Input: part model. Units: mm. Frame: model coordinates. Coordinates: 2 decimals unless noted, no trailing zeros. Order: outer loops, then holes, each group sorted by start corner. A loop starts at its lowest first (then second) coordinate and runs counter-clockwise, first axis right, second up. Notation, with made-up numbers: (23, -34) -> (29, -34) arc R34 cw to (29, 4) -> close; hole circle Ø8 at (-10, -23). An arc over 180 degrees is marked (long way). Answer as CSV lines item,"result".
from build123d import *

# Parameters (mm, degrees)
SKETCH1_W               = 225.298
SKETCH1_H               = 399.796
BOSS_EXTRUDE1_DEPTH     = 6.35
SKETCH2_R               = 14.351
CUT_EXTRUDE1_DEPTH      = 1
CUT_EXTRUDE1_DEPTH_BACK = 7.35


with BuildPart() as part:
    # Sketch1 → Boss-Extrude1 (new body)
    with BuildSketch(Plane(origin=(0, 0, 0), x_dir=(0, 0, -1), z_dir=(1, 0, 0))):
        with Locations((112.649, 199.898)):
            Rectangle(SKETCH1_W, SKETCH1_H)
    extrude(amount=BOSS_EXTRUDE1_DEPTH)

    # Sketch2 → Cut-Extrude1 (cut, two sides)
    with BuildSketch(Plane(origin=(6.35, 0, 0), x_dir=(0, 0, -1), z_dir=(1, 0, 0))) as cut_extrude1_sk:
        with Locations((199.898, 199.898)):
            Circle(SKETCH2_R)
    extrude(amount=CUT_EXTRUDE1_DEPTH, mode=Mode.SUBTRACT)
    extrude(cut_extrude1_sk.sketch, amount=-CUT_EXTRUDE1_DEPTH_BACK, mode=Mode.SUBTRACT)


solid = part.part
1. Ray query, line 1 along Z through (x, y) = (3, 189). Return the intervals inside material, ascending.
Findings:
line 1,"z = -225.3 to -209.24, -190.56 to 0"
2. Cut plane A-A (z = -193.5). Return the cut outline in (x, y), plus the area to 3 significant figures.
Findings:
outline,"(0, 0) -> (6.35, 0) -> (6.35, 187.05) -> (0, 187.05) -> close; (0, 212.74) -> (6.35, 212.74) -> (6.35, 399.8) -> (0, 399.8) -> close"
area,"2,380 mm2"
3. Mould query, pull axis Y, two halves, no side actions, for faces 1 (the face through (6.35, 203, -111)), 2 (the face through (3.219, 214.127, -198.03)). Classes: released by +Y, released by -Y, zero draft, split by the parting line, or undercut.
Findings:
face 1,"zero draft"
face 2,"undercut"
